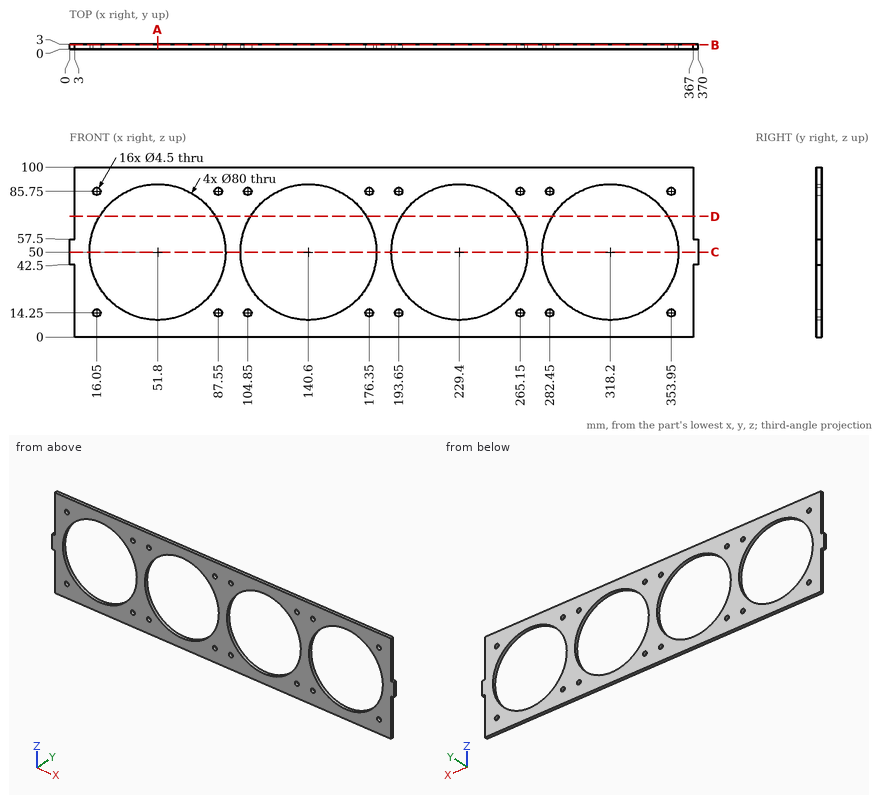
Input: dimensioned drawing with shaded views. Units: mm. Origin: part minimum x, y, z. Give positions to 0.01 mm unless a question says otherwise; leave off trailing zeros. Write each loop counter-clockwise with the first axis right and the second up, starting at its lowest first coordinate (ties: lowest second). Pieces come first, ordered by that corner, then holes. Notation, with made-up numbers: (5, -32.5) - (14, -32.5) arc R22 cw to (14, -0.5) - close; hole circle Ø8 at (38.5, -39). An arc over 180 degrees is marked (long way). Write item = value, one per line. Start each with the question number.
1) Cut plane D-D (z = 71). Return loops of the section in (x, y), and give its area (3 significant figures).
2) Cut plane A-A (x = 51.8). Return loops of the section in (y, z).
3) Material intervals for L1, parallel to Z at x = 282.45, y = 2.3; L2, parallel to X at y = 1.1, z = 56.5; L3, parallel to X at y = 0.35, z = 91.5, sorted ascending. Write a range as [from, to].
4) Cut plane C-C (z = 50). Return loops of the section in (x, y), and give its area (3 significant figures).
5) Cut plane B-B (y = 2.45). Give the number of separate pieces and of enclosed holes in the cut face, and give its area (3 significant figures).
6) Pin query (flat end, axial travel): pin 1 (1.5 mm diameter, centred on y = 1, z = 83, fed in from +X); pin 2 (7 mm diameter, centred on x = 193.65, z = 14.25, fed in from -Y); pin 3 (1.5 mm diameter, centred on y = 1, z = 89.5, fed in from -X). Return the tip coordinate at first contact, or that it passes through.
Answers follow:
q1.outline = (3, 0) - (17.76, 0) - (17.76, 3) - (3, 3) - close; (85.84, 0) - (106.56, 0) - (106.56, 3) - (85.84, 3) - close; (174.64, 0) - (195.36, 0) - (195.36, 3) - (174.64, 3) - close; (263.44, 0) - (284.16, 0) - (284.16, 3) - (263.44, 3) - close; (352.24, 0) - (367, 0) - (367, 3) - (352.24, 3) - close
q1.area = 275 mm^2
q2.outline = (0, 0) - (3, 0) - (3, 10) - (0, 10) - close; (0, 90) - (3, 90) - (3, 100) - (0, 100) - close
q3.L1 = [0, 12], [16.5, 32.06], [67.94, 83.5], [88, 100]
q3.L2 = [0, 12.33], [91.27, 101.13], [180.07, 189.93], [268.87, 278.73], [357.67, 370]
q3.L3 = [3, 367]
q4.outline = (0, 0) - (11.8, 0) - (11.8, 3) - (0, 3) - close; (91.8, 0) - (100.6, 0) - (100.6, 3) - (91.8, 3) - close; (180.6, 0) - (189.4, 0) - (189.4, 3) - (180.6, 3) - close; (269.4, 0) - (278.2, 0) - (278.2, 3) - (269.4, 3) - close; (358.2, 0) - (370, 0) - (370, 3) - (358.2, 3) - close
q4.area = 150 mm^2
q5.separate_pieces = 1
q5.enclosed_holes = 20
q5.area = 16,100 mm^2
q6.pin_1 = 367
q6.pin_2 = 0
q6.pin_3 = 3
